Geometry check sheet. Reference: the model listing, model coordinates, mm. Coordinates: 2 decimals unless noted, no trailing zeros. Write each loop counter-clockwise with the first axis right and the second up, starting at its lowest first coordinate (ties: lowest second). Pieces come first, ordered by that corner, then holes. Notation, with made-up numbers: M 19.5,-30 L 27.5,-30 A13 ccw 27.5,-16 Z; hole C -26.5,86.25 d11. An arc over 180 degrees is marked long. Write each question's results on one line, items separated by ' | '.
```python
from build123d import *

# Parameters (mm, degrees)
SKETCH_1_W          = 250
SKETCH_1_H          = 370
EXTRUDE_1_DEPTH     = 20
CHAMFER_1_SIZE      = 8
SKETCH_2_W          = 230
SKETCH_2_H          = 350
SKETCH_2_W_2        = 210
SKETCH_2_H_2        = 330
CUT_EXTRUDE_1_DEPTH = 10


with BuildPart() as part:
    # Эскиз1 → Бобышка-Вытянуть1 (new body)
    with BuildSketch(Plane.XY):
        Rectangle(SKETCH_1_W, SKETCH_1_H)
    extrude(amount=EXTRUDE_1_DEPTH)

    # Фаска1
    chamfer_1_edges = [part.edges().sort_by_distance(p)[0] for p in [
        (0, -185, 20),
        (-125, 0, 20),
        (0, 185, 20),
        (125, 0, 20),
    ]]
    chamfer(chamfer_1_edges, length=CHAMFER_1_SIZE)

    # Эскиз2 → Вырез-Вытянуть1 (cut)
    with BuildSketch(Plane.XY.offset(20)):
        Rectangle(SKETCH_2_W, SKETCH_2_H)
        Rectangle(SKETCH_2_W_2, SKETCH_2_H_2, mode=Mode.SUBTRACT)
    extrude(amount=-CUT_EXTRUDE_1_DEPTH, mode=Mode.SUBTRACT)


solid = part.part
```
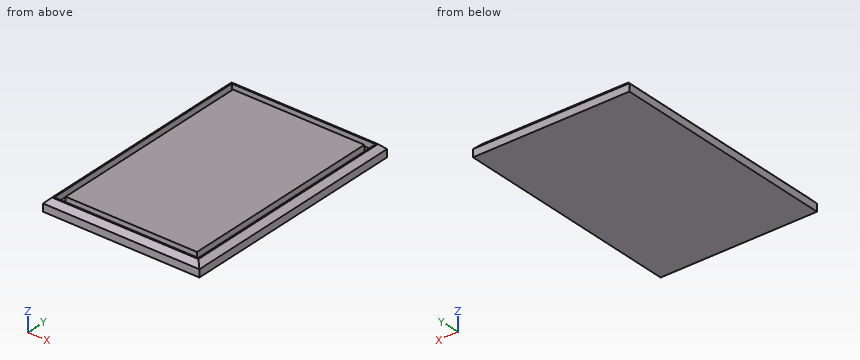
Q1. Scan lines: probe 1 along X at (y, z) = (139.5, 11.5); probe 2 along Y at (x, z) = (-69, 15.5); probe 3 along X at (y, z) = (121, 15). Record each from-to range of solid material in increasing order.
Geometry check:
probe 1: x = -125 to -115, -105 to 105, 115 to 125 | probe 2: y = -181.5 to -175, -165 to 165, 175 to 181.5 | probe 3: x = -122 to -115, -105 to 105, 115 to 122
Q2. Sectioned sample at C-C on x = -35.5. Record the cut outline in (y, z), and give its area (3 significant figures).
Geometry check:
outline: M -185,0 L 185,0 L 185,12 L 177,20 L 175,20 L 175,10 L 165,10 L 165,20 L -165,20 L -165,10 L -175,10 L -175,20 L -177,20 L -185,12 Z | area: 7,140 mm2
Q3. Sectioned sample at B-B on y = -72.5. Record the cut outline in (x, z).
Geometry check:
outline: M -125,0 L 125,0 L 125,12 L 117,20 L 115,20 L 115,10 L 105,10 L 105,20 L -105,20 L -105,10 L -115,10 L -115,20 L -117,20 L -125,12 Z
Q4. Depth check by flat-ended pin: P1, Ø3, axis at y = -62, z = 16, coming from the -X side; P2, Ø3, axis at x = -34.5, z = 17, coming from the -Y side; P3, Ø5, axis at y = -38, z = 16, coming from the +X side. Enter the tip coordinate at first touch or a pass-through.
Geometry check:
P1: stops at x = -122.5 | P2: stops at y = -181.5 | P3: stops at x = 123.5
Q5. Sectioned sample at A-A on z = 16.75. Record the cut outline in (x, y).
Geometry check:
outline: M -120.25,-180.25 L 120.25,-180.25 L 120.25,180.25 L -120.25,180.25 Z; M -105,-165 L 105,-165 L 105,165 L -105,165 Z; hole M -115,-175 L 115,-175 L 115,175 L -115,175 Z
